Build history of the part. All positions in model axes, mm. A direction names the side the tool comes from. Round coordinates to 2 decimals unless told otherwise and drop trailing zeros. Write each loop counter-clockwise with the first axis right and the second up, starting at its lowest first coordinate (ties: lowest second). Pieces come first, ordered by that corner, then holes.
1) Wall check: probe 1 along Y at (x, z) = (169.5, 2.25); probe 2 along X at (y, z) = (64, 1.25); probe 3 along Y at (x, z) = (45.5, 1.3). Give the ranges that are in metal, low to high.
2) Saw through at A-A (y = 69.5). Write the cut outline in (x, z), plus the area to 4 significant figures.
3) Saw through at B-B (x = 191). Write the cut outline in (y, z), plus the area to 4 significant figures.
4) Saw through at D-D (x = 148.5). Write the cut outline in (y, z).
5) Saw through at C-C (z = -0.8). State how many separate pieces and enclosed holes the cut face has, plus the area to 3 significant figures.
6) Pull direction X, two halves, no side cores. Call faces 1 (the cylindrical face through (46.995, 42.272, 0.465)), 2 (the flat face through (48, 53, -2)), 3 (the cylindrical face through (203.46, 28.32, -0.99)): +X half, -X half, draft (parallel to the pull), parting line (faces both ways), or undercut.
7) Which spindle directions (+Z, -Z, +X, -X, +Y, -Y) get a long thin tool onto all of the face, cutting with end or side? Do faces 4 (the flat face through (128.8, 49.08, 1.48)), 5 (the flat face through (165, 53, -2)), 6 (the cylindrical face through (162.435, 44.201, -1.014)). Say none if no direction does.
8) Flat gauge pins, fed straight in: pin 1 (2.5 mm diameter, centred on x = 169.5, y = 64, fed in from -Z); pin 2 (1.5 mm diameter, centred on x = 113, y = 19, fed in from -Z). Where does each tip first touch, or does it go through?
from build123d import *
from OCP.BRepFilletAPI import BRepFilletAPI_MakeChamfer

# Parameters (mm, degrees)
SZKIC1_W                    = 215
SZKIC1_H                    = 93
DODANIE_WYCI_GNI_CIE1_DEPTH = 3
DODANIE_WYCI_GNI_CIE3_DEPTH = 5
SZKIC4_R                    = 1.9
WYTNIJ_WYCI_GNI_CIE1_DEPTH  = 10
SZKIC5_R                    = 1.9
SZKIC5_W                    = 117.5
SZKIC5_H                    = 28
WYTNIJ_WYCI_GNI_CIE2_DEPTH  = 35
SFAZOWANIE1_SIZE            = 2
SFAZOWANIE1_SIZE2           = 1.42483793
SFAZOWANIE1_SIZE2_2         = 2.349845037
SZKIC6_R                    = 10.75
SZKIC6_R_2                  = 1.9
SZKIC6_R_3                  = 2
SZKIC6_W                    = 13.5
SZKIC6_H                    = 6
WYTNIJ_WYCI_GNI_CIE3_DEPTH  = 238.314137801
SZKIC8_R                    = 3.5
SZKIC8_R_2                  = 2
DODANIE_WYCI_GNI_CIE4_DEPTH = 2
SZKIC9_R                    = 1.9
WYTNIJ_WYCI_GNI_CIE4_DEPTH  = 3
DODANIE_WYCI_GNI_CIE5_START = 2
SZKIC10_R                   = 4
SZKIC10_R_2                 = 1.9
DODANIE_WYCI_GNI_CIE5_DEPTH = 2
SZKIC11_R                   = 8.25
WYTNIJ_WYCI_GNI_CIE5_DEPTH  = 10
CUT_EXTRUDE1_REACH          = 152.101


with BuildPart() as part:
    # Szkic1 → Dodanie-wyciągnięcie1 (new body)
    with BuildSketch(Plane.XY):
        with Locations((107.5, 46.5)):
            Rectangle(SZKIC1_W, SZKIC1_H)
    extrude(amount=DODANIE_WYCI_GNI_CIE1_DEPTH)

    # Szkic3 → Dodanie-wyciągnięcie3 (add, symmetric)
    with BuildSketch(Plane(origin=(107.5, 0, 0), x_dir=(0, 0, -1), z_dir=(1, 0, 0))):
        Polygon((0, 3), (10, 3), (35, 35), (35, 41), (0, 41), align=None)
        Polygon((3, 11.541451884), (3, 35), (31.193011155, 35), (9.799205499, 7.615928759), align=None, mode=Mode.SUBTRACT)
    extrude(amount=DODANIE_WYCI_GNI_CIE3_DEPTH, both=True)

    # Szkic4 → Wytnij-wyciągnięcie1 (cut)
    with BuildSketch(Plane.XZ.offset(-3)):
        with Locations(Location((107.5, -5, 0), (0, 0, 270))):
            Circle(SZKIC4_R)
    extrude(amount=-WYTNIJ_WYCI_GNI_CIE1_DEPTH, mode=Mode.SUBTRACT)

    # Szkic5 → Wytnij-wyciągnięcie2 (cut)
    with BuildSketch(Plane.XY.offset(3)):
        with Locations((45.5, 84)):
            Circle(SZKIC5_R)
        with Locations((45.5, 64)):
            Circle(SZKIC5_R)
        with Locations((169.5, 64)):
            Circle(SZKIC5_R)
        with Locations((169.5, 84)):
            Circle(SZKIC5_R)
        with Locations((107.5, 74)):
            Rectangle(SZKIC5_W, SZKIC5_H)
    extrude(amount=-WYTNIJ_WYCI_GNI_CIE2_DEPTH, mode=Mode.SUBTRACT)

    # Sfazowanie1: one chamfer whose edges measure the first distance from different faces: ONE call of the kernel's chamfer builder (chamfer() names one face for all edges)
    sfazowanie1_edges_1 = [part.edges().sort_by_distance(p)[0] for p in [
        (107.5, 35, -31.193011155),
    ]]
    sfazowanie1_side_1 = [part.faces().sort_by_distance(p)[0] for p in [
        (107.5, 35, -17.096505578),
    ]]
    sfazowanie1_edges_2 = [part.edges().sort_by_distance(p)[0] for p in [
        (107.5, 35, -3),
    ]]
    sfazowanie1_edges_3 = [part.edges().sort_by_distance(p)[0] for p in [
        (107.5, 7.615928759, -9.799205499),
    ]]
    sfazowanie1_side_3 = [part.faces().sort_by_distance(p)[0] for p in [
        (107.5, 21.30796438, -20.496108327),
    ]]
    sfazowanie1 = BRepFilletAPI_MakeChamfer(part.part.solid().wrapped)
    for e in sfazowanie1_edges_1:
        sfazowanie1.Add(SFAZOWANIE1_SIZE, SFAZOWANIE1_SIZE2, e.wrapped, sfazowanie1_side_1[0].wrapped)  # the first distance lies on this face
    for e in sfazowanie1_edges_2:
        sfazowanie1.Add(SFAZOWANIE1_SIZE, e.wrapped)
    for e in sfazowanie1_edges_3:
        sfazowanie1.Add(SFAZOWANIE1_SIZE, SFAZOWANIE1_SIZE2_2, e.wrapped, sfazowanie1_side_3[0].wrapped)  # the first distance lies on this face
    add(Compound.cast(sfazowanie1.Shape()), mode=Mode.REPLACE)

    # Szkic6 → Wytnij-wyciągnięcie3 (cut, through all)
    with BuildSketch(Plane.XY.offset(3)):
        with Locations((191, 15.35)):
            Circle(SZKIC6_R)
        with Locations((203, 24.85)):
            Circle(SZKIC6_R_2)
        with Locations((179, 5.85)):
            Circle(SZKIC6_R_2)
        with Locations((148.5, 25.05)):
            Circle(SZKIC6_R_3)
        with Locations((169.25, 25.05)):
            Circle(SZKIC6_R_3)
        with Locations((160.25, 7.8)):
            Rectangle(SZKIC6_W, SZKIC6_H)
        with BuildLine():
            Line((167, 20.8), (153.9, 20.8))
            ThreePointArc((153.9, 20.8), (151.849390335, 21.649390335), (151, 23.7))
            Line((151, 23.7), (151, 26.4))
            ThreePointArc((151, 26.4), (151.849390335, 28.450609665), (153.9, 29.3))
            Line((153.9, 29.3), (167, 29.3))
            Line((167, 29.3), (167, 20.8))
        make_face()
    extrude(amount=-WYTNIJ_WYCI_GNI_CIE3_DEPTH, mode=Mode.SUBTRACT)

    # Szkic8 → Dodanie-wyciągnięcie4 (add)
    # profile 1 of 2: a face of its own
    with BuildSketch(Plane(origin=(0, 0, 0), x_dir=(-1, 0, 0), z_dir=(0, 0, -1))):
        with Locations((-179, 5.85)):
            Circle(SZKIC8_R)
        with Locations((-179, 5.85)):
            Circle(SZKIC8_R_2, mode=Mode.SUBTRACT)
    # profile 2 of 2: a face of its own
    with BuildSketch(Plane(origin=(0, 0, 0), x_dir=(-1, 0, 0), z_dir=(0, 0, -1))):
        with Locations((-203, 24.85)):
            Circle(SZKIC8_R)
        with Locations((-203, 24.85)):
            Circle(SZKIC8_R_2, mode=Mode.SUBTRACT)
    extrude(amount=DODANIE_WYCI_GNI_CIE4_DEPTH)

    # Szkic9 → Wytnij-wyciągnięcie4 (cut)
    with BuildSketch(Plane(origin=(0, 0, 0), x_dir=(-1, 0, 0), z_dir=(0, 0, -1))):
        with BuildLine():
            Line((-150.385024789, 55), (-156.25, 55))
            ThreePointArc((-156.25, 55), (-162.25, 49), (-156.25, 43))
            Line((-156.25, 43), (-150.385024789, 55))
        make_face()
        Polygon((-140.144746897, 55), (-146.385024789, 55), (-152.25, 43), (-146.009722108, 43), align=None)
        Polygon((-129.904469005, 55), (-136.144746897, 55), (-142.009722108, 43), (-135.769444216, 43), align=None)
        Polygon((-119.664191113, 55), (-125.904469005, 55), (-131.769444216, 43), (-125.529166324, 43), align=None)
        Polygon((-109.423913221, 55), (-115.664191113, 55), (-121.529166324, 43), (-115.288888432, 43), align=None)
        Polygon((-99.183635329, 55), (-105.423913221, 55), (-111.288888432, 43), (-105.04861054, 43), align=None)
        Polygon((-88.943357437, 55), (-95.183635329, 55), (-101.04861054, 43), (-94.808332648, 43), align=None)
        Polygon((-78.703079545, 55), (-84.943357437, 55), (-90.808332648, 43), (-84.568054757, 43), align=None)
        Polygon((-68.462801653, 55), (-74.703079545, 55), (-80.568054757, 43), (-74.327776865, 43), align=None)
        with BuildLine():
            Line((-58.75, 55), (-64.462801653, 55))
            Line((-64.462801653, 55), (-70.327776865, 43))
            Line((-70.327776865, 43), (-64.087498973, 43))
            Line((-64.087498973, 43), (-58.233413005, 54.977720124))
            ThreePointArc((-58.233413005, 54.977720124), (-58.491466387, 54.994427443), (-58.75, 55))
        make_face()
        with BuildLine():
            Line((-54.904147181, 53.605368183), (-60.087498973, 43))
            Line((-60.087498973, 43), (-58.75, 43))
            ThreePointArc((-58.75, 43), (-53.109423385, 46.954542728), (-54.904147181, 53.605368183))
        make_face()
        with Locations((-166.25, 55)):
            Circle(SZKIC9_R)
        with Locations((-166.25, 43)):
            Circle(SZKIC9_R)
        with Locations((-48.75, 43)):
            Circle(SZKIC9_R)
        with Locations((-48.75, 55)):
            Circle(SZKIC9_R)
    extrude(amount=-WYTNIJ_WYCI_GNI_CIE4_DEPTH, mode=Mode.SUBTRACT)

    # Szkic10 → Dodanie-wyciągnięcie5 (add)
    # profile 1 of 4: a face of its own
    with BuildSketch(Plane(origin=(0, 0, 0), x_dir=(-1, 0, 0), z_dir=(0, 0, -1)).offset(DODANIE_WYCI_GNI_CIE5_START)):
        with Locations((-166.25, 55)):
            Circle(SZKIC10_R)
        with Locations((-166.25, 55)):
            Circle(SZKIC10_R_2, mode=Mode.SUBTRACT)
    # profile 2 of 4: a face of its own
    with BuildSketch(Plane(origin=(0, 0, 0), x_dir=(-1, 0, 0), z_dir=(0, 0, -1)).offset(DODANIE_WYCI_GNI_CIE5_START)):
        with Locations((-166.25, 43)):
            Circle(SZKIC10_R)
        with Locations((-166.25, 43)):
            Circle(SZKIC10_R_2, mode=Mode.SUBTRACT)
    # profile 3 of 4: a face of its own
    with BuildSketch(Plane(origin=(0, 0, 0), x_dir=(-1, 0, 0), z_dir=(0, 0, -1)).offset(DODANIE_WYCI_GNI_CIE5_START)):
        with Locations((-48.75, 43)):
            Circle(SZKIC10_R)
        with Locations((-48.75, 43)):
            Circle(SZKIC10_R_2, mode=Mode.SUBTRACT)
    # profile 4 of 4: a face of its own
    with BuildSketch(Plane(origin=(0, 0, 0), x_dir=(-1, 0, 0), z_dir=(0, 0, -1)).offset(DODANIE_WYCI_GNI_CIE5_START)):
        with Locations((-48.75, 55)):
            Circle(SZKIC10_R)
        with Locations((-48.75, 55)):
            Circle(SZKIC10_R_2, mode=Mode.SUBTRACT)
    extrude(amount=-DODANIE_WYCI_GNI_CIE5_DEPTH)

    # Szkic11 → Wytnij-wyciągnięcie5 (cut)
    with BuildSketch(Plane(origin=(0, 0, 0), x_dir=(-1, 0, 0), z_dir=(0, 0, -1))):
        with Locations((-129.5, 15.8)):
            Circle(SZKIC11_R)
    extrude(amount=-WYTNIJ_WYCI_GNI_CIE5_DEPTH, mode=Mode.SUBTRACT)

    # Sketch1 → Cut-Extrude1 (cut, up to next)
    with BuildSketch(Plane(origin=(112.5, 0, 0), x_dir=(0, 0, -1), z_dir=(1, 0, 0)), mode=Mode.PRIVATE) as cut_extrude1_sk1:
        Polygon((0, 41), (0, 3), (10, 3), (35, 35), (35, 41), align=None)
    cut_extrude1_tool1 = extrude(cut_extrude1_sk1.sketch, amount=-CUT_EXTRUDE1_REACH, mode=Mode.PRIVATE) & part.part
    add(cut_extrude1_tool1.solids().sort_by_distance((112.5, 25.584229, -13.557348))[0], mode=Mode.SUBTRACT)


solid = part.part
Evaluation:
1. probe 1: y = 0 to 23.07, 27.03 to 62.1, 65.9 to 82.1, 85.9 to 93
1. probe 2: x = 0 to 43.6, 47.4 to 48.75, 166.25 to 167.6, 171.4 to 215
1. probe 3: y = 0 to 62.1, 65.9 to 82.1, 85.9 to 93
2. outline: (0, 0) - (48.75, 0) - (48.75, 3) - (0, 3) - close; (166.25, 0) - (215, 0) - (215, 3) - (166.25, 3) - close
2. area: 292.5 mm2
3. outline: (0, 0) - (4.6, 0) - (4.6, 3) - (0, 3) - close; (26.1, 0) - (93, 0) - (93, 3) - (26.1, 3) - close
3. area: 214.5 mm2
4. outline: (0, 0) - (23.05, 0) - (23.05, 3) - (0, 3) - close; (27.05, 0) - (43, 0) - (43, 3) - (27.05, 3) - close; (50.67, 0) - (60, 0) - (60, 3) - (50.67, 3) - close; (88, 0) - (93, 0) - (93, 3) - (88, 3) - close
5. separate pieces: 6
5. enclosed holes: 6
5. area: 208 mm2
6. face 1: undercut
6. face 2: draft
6. face 3: parting line
7. face 4: +Z, -Z
7. face 5: -Z, +X, -X, +Y, -Y
7. face 6: -Z
8. pin 1: passes through
8. pin 2: stops at z = 0
